Autodesk Inventor part; units mm, degrees
ref_plane "YZ Plane" through (0, 0, 0) normal (1, 0, 0) x (0, 1, 0)
ref_plane "XZ Plane" through (0, 0, 0) normal (0, 1, 0) x (-1, 0, 0)
ref_plane "XY Plane" through (0, 0, 0) normal (0, 0, 1) x (1, 0, 0)
sketch "Sketch1" plane through (0, 0, 0) normal (0, 0, 1) x (1, 0, 0)
  line L0 (0, 0) -> (2.9424, 0)
  line L1 (2.9424, 0) -> (2.9424, -7.2806)
  line L2 (2.9424, -7.2806) -> (0, -7.2806)
  line L3 (0, -7.2806) -> (0, 0)
extrude "Extrusion1" add sketch "Sketch1" along normal blind 25.4
sketch "Sketch2" plane through (2.9424, -7.2806, 0) normal (1, 0, 0) x (0, 0, -1)
  point P0 (0, 7.2806)
sketch "Sketch3" plane through (2.9424, -7.2806, 0) normal (1, 0, 0) x (0, 0, -1)
  line L0 (-9.1297, 6.2288) -> (-14.2174, 6.2288)
  line L1 (-14.2174, 6.2288) -> (-14.2174, 0.7246)
  line L2 (-14.2174, 0.7246) -> (-9.1297, 0.7246)
  line L3 (-9.1297, 0.7246) -> (-9.1297, 6.2288)
  point P0 (0, 7.2806)
extrude "Extrusion2" add sketch "Sketch3" along normal blind 2.032
fillet "Fillet1" radius 1.27 3 edges at (4.9744, -1.0519, 11.6735) (4.9744, -6.556, 11.6735) (2.9424, -1.0519, 11.6735)
sketch "Sketch4" plane through (4.9744, -7.2806, 0) normal (1, 0, 0) x (0, 0, -1)
  line L0 (-12.9198, 2.186) -> (-11.0597, 2.186)
  line L1 (-11.0597, 2.186) -> (-11.0597, 4.7902)
  line L2 (-11.0597, 4.7902) -> (-12.9198, 4.7902)
  line L3 (-12.9198, 4.7902) -> (-12.9198, 2.186)
  point P0 (0, 7.2806)
extrude "Extrusion3" add sketch "Sketch4" along normal blind 2.286
sketch "Sketch5" plane through (4.9744, -7.2806, 0) normal (1, 0, 0) x (0, 0, -1)
  point P0 (0, 7.2806)
sketch "Sketch6" plane through (7.2604, -3.8837, 11.7408) normal (1, 0, 0) x (0, 0, -1)
  point P0 (11.7408, 3.8837)
sketch "Sketch7" plane through (4.9744, -5.0946, 12.9198) normal (0, 0, 1) x (1, 0, 0)
  circle A0 centre (1.0916, 1.297) radius 0.6417
  point P0 (-4.9744, 5.0946)
extrude "Extrusion4" cut sketch "Sketch7" against normal blind 25.4
sketch "Sketch8" plane through (0, -7.2806, 0) normal (0, -1, 0) x (1, 0, 0)
  point P0 (0, 0)
sketch "Sketch9" plane through (0, -7.2806, 0) normal (-1, 0, 0) x (0, 0, 1)
  line L0 (8.6535, 6.5442) -> (10.8988, 6.5442)
  line L1 (10.8988, 6.5442) -> (10.8988, 5.8257)
  line L2 (10.8988, 5.8257) -> (8.6535, 5.8257)
  line L3 (8.6535, 5.8257) -> (8.6535, 6.5442)
  point P0 (0, 7.2806)
extrude "Extrusion5" add sketch "Sketch9" along normal blind 1.778
sketch "Sketch10" plane through (0, -7.2806, 0) normal (-1, 0, 0) x (0, 0, 1)
  line L0 (9.1297, 1.9946) -> (14.2174, 1.9946)
  line L1 (8.5112, 2.6437) -> (10.4941, 2.6437)
  line L2 (10.4941, 2.6437) -> (10.4941, 1.9946)
  line L3 (10.4941, 1.9946) -> (8.5112, 1.9946)
  line L4 (8.5112, 1.9946) -> (8.5112, 2.6437)
  point P0 (0, 7.2806)
extrude "Extrusion6" add sketch "Sketch10" along normal blind 1.778
properties part number "pen holder" material "Wood (Oak)"
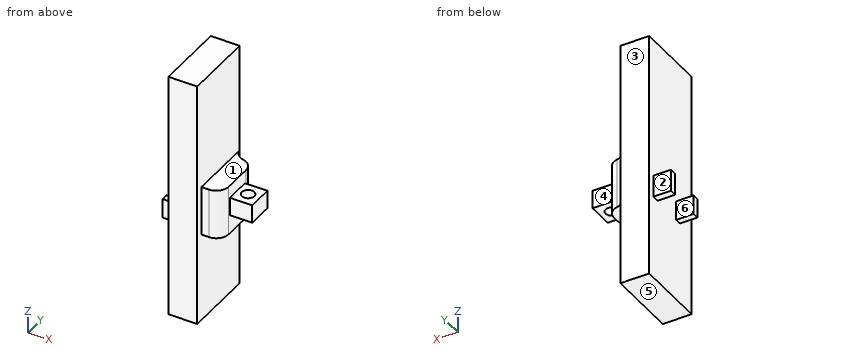
Model file for the job. Use its own axes, mm. Face numbers are marked on the shaded views. A direction names the side the tool comes from. Give positions to 0.01 mm unless a question says otherwise; leave off trailing zeros. Order: outer loops, then holes, each group sorted by start corner. A loop starts at its lowest first (then second) coordinate and runs counter-clockwise, first axis right, second up.
1) Wall check: probe 1 along X at (y, z) = (-2.25, 8); probe 2 along Z at (x, y) = (3.5, -4.75); probe 3 along X at (y, z) = (-5.25, 13). Give the ranges that are in metal, low to high.
2) 3-axis set-ups, long thin cutter, end or side, ignore diameter. For the marked faces 1, 2 and 3: which of +Z, -Z, +X, -X, +Y, -Y reach the whole face in a straight line?
3) Pin check, flat tips, straight feed: pin 1 (0.5 mm diameter, centred on x = -1, z = 10, fed in from -Y); pin 2 (0.5 mm diameter, centred on x = -0.5, y = -5, fed in from -Z); pin 3 (3 mm diameter, centred on y = -3.5, z = 23, fed in from +X); pin 4 (1 mm diameter, centred on x = 6, z = 8, fed in from +Y). Stop position of each tip, or through.
4) Saw through at D-D, the plane z = 19.5. Write the cut outline in (x, y), then the cut area to 3 significant figures.
5) Saw through at C-C, the plane x = 4.75. Write the cut outline in (y, z).
6) Mould opens along Y. For the marked faces 4, 5 and 6 say: +Y half, -Y half, draft (parallel to the pull), parting line (faces both ways), or undercut.
7) Saw through at A-A, the plane z = 12.5. Write the cut outline in (x, y).
8) Saw through at B-B, the plane y = -5.75. Write the cut outline in (x, z).
Computed:
1. probe 1: x = 0 to 2.94
1. probe 2: z = 9.13 to 14.22
1. probe 3: x = 0 to 4.97
2. face 1: +Z, +X, +Y, -Y
2. face 2: +Z, -Z, -X, +Y
2. face 3: +Z, -Z, +X, -X, +Y
3. pin 1: stops at y = -5.29
3. pin 2: stops at z = 8.51
3. pin 3: stops at x = 2.94
3. pin 4: passes through
4. outline: (0, -7.28) - (2.94, -7.28) - (2.94, 0) - (0, 0) - close
4. area: 21.4 mm2
5. outline: (-6.01, 9.13) - (-1.6, 9.13) - (-1.6, 14.22) - (-6.01, 14.22) - close
6. face 4: +Y half
6. face 5: draft
6. face 6: undercut
7. outline: (0, -7.28) - (2.94, -7.28) - (2.94, -6.56) - (3.7, -6.56) arc R1.27 ccw to (4.97, -5.29) - (4.97, -5.09) - (7.26, -5.09) - (7.26, -2.49) - (4.97, -2.49) - (4.97, -2.32) arc R1.27 ccw to (3.95, -1.08) arc R1.27 cw to (2.94, 0) - (0, 0) - close; hole circle Ø1.28 at (6.07, -3.8)
8. outline: (0, 0) - (2.94, 0) - (2.94, 9.13) - (4.89, 9.13) - (4.89, 14.22) - (2.94, 14.22) - (2.94, 25.4) - (0, 25.4) - close
